from build123d import *

# Parameters (mm, degrees)
F0_R         = 15
F1_DEPTH     = 74
F2_R         = 15
F2_R_2       = 9.975
F3_DEPTH     = 3
F4_R         = 15
F4_R_2       = 10.0175
F5_DEPTH     = 22
F6_R         = 15
F6_R_2       = 7.5
F7_DEPTH     = 19
F8_SIZE2     = 1
F8_SIZE      = 1
F12_DEPTH    = 26.5
F13_T1_DEPTH = 5
F16_DEPTH    = 3


# Not quite as in the source:
# - a fillet or chamfer that OpenCascade refuses, or shapes differently, is made with other operations: its cross-section is extruded or revolved along the edge and cut away or added


with BuildPart() as f1:
    # F0 (on Front) → F1 (new body)
    with BuildSketch(Plane.XZ):
        Circle(F0_R)
    extrude(amount=F1_DEPTH)

    # F2 (on face) → F3 (cut)
    with BuildSketch(Plane.XZ.offset(74)):
        Circle(F2_R)
        Circle(F2_R_2, mode=Mode.SUBTRACT)
    extrude(amount=-F3_DEPTH, mode=Mode.SUBTRACT)

    # F4 (on face) → F5 (cut)
    with BuildSketch(Plane.XZ.offset(71)):
        Circle(F4_R)
        Circle(F4_R_2, mode=Mode.SUBTRACT)
    extrude(amount=-F5_DEPTH, mode=Mode.SUBTRACT)

    # F6 (on Front) → F7 (cut)
    with BuildSketch(Plane.XZ):
        Circle(F6_R)
        Circle(F6_R_2, mode=Mode.SUBTRACT)
    extrude(amount=F7_DEPTH, mode=Mode.SUBTRACT)

    # F8
    f8_edges = [f1.edges().sort_by_distance(p)[0] for p in [
        (-7.5, 0, 0),
        (-9.975, -74, 0),
    ]]
    chamfer(f8_edges, length=F8_SIZE, length2=F8_SIZE2)

    # F9 (on Right) → F10 (revolve, cut)
    with BuildSketch(Plane.YZ):
        Polygon((-26.5, 15), (-19, 7.5), (-19, 15), align=None)
    revolve(axis=Axis((0, -22.75, 0), (0, 1, 0)), mode=Mode.SUBTRACT)

    # F11 (on face) → F12 (cut)
    with BuildSketch(Plane.XZ.offset(74)):
        with BuildLine():
            Line((-2.5, 14.7901994577), (-2.5, 10.0175))
            Line((-2.5, 10.0175), (-2.5, 9.0175))
            Line((-2.5, 9.0175), (0, 9.0175))
            Line((0, 9.0175), (2.5, 9.0175))
            Line((2.5, 9.0175), (2.5, 10.0175))
            Line((2.5, 10.0175), (2.5, 14.7901994577))
            ThreePointArc((2.5, 14.7901994577), (0, 15), (-2.5, 14.7901994577))
        make_face()
    extrude(amount=-F12_DEPTH, mode=Mode.SUBTRACT)

    # F13: fillet of radius 2.5 on 1 edges, made by hand

    # F13_s2 → F13_t1 (join)
    with BuildSketch(Plane.YZ.offset(-2.5)):
        with BuildLine():
            add(Edge.make_bspline(
                [(-50, 9.0175), (-47.5, 9.0175), (-47.5, 11.5175)],
                knots=[0, 0, 0, 1, 1, 1], degree=2, weights=[1, 1, 1]))
            Line((-47.5, 11.5175), (-47.45, 11.5175))
            Line((-47.45, 11.5175), (-47.45, 8.9675))
            Line((-47.45, 8.9675), (-50, 8.9675))
            Line((-50, 8.9675), (-50, 9.0175))
        make_face()
    extrude(amount=F13_T1_DEPTH)

    # F15 (on offset) → F16 (cut)
    with BuildSketch(Plane.XY.offset(7.5)):
        with BuildLine():
            Line((2.5, -9), (2.5, -4))
            ThreePointArc((2.5, -4), (1.767766953, -2.232233047), (0, -1.5))
            ThreePointArc((0, -1.5), (-1.767766953, -2.232233047), (-2.5, -4))
            Line((-2.5, -4), (-2.5, -9))
            ThreePointArc((-2.5, -9), (-1.767766953, -10.767766953), (0, -11.5))
            ThreePointArc((0, -11.5), (1.767766953, -10.767766953), (2.5, -9))
        make_face()
    extrude(amount=-F16_DEPTH, mode=Mode.SUBTRACT)


solid = f1.part
Model file for the job. Use its own axes, mm. A direction names the side the tool comes from. Give positions to 0.01 mm unless a question says otherwise; leave off trailing zeros. Order: outer loops, then holes, each group sorted by start corner. A loop starts at its lowest first (then second) coordinate and runs counter-clockwise, first axis right, second up. Notation, with made-up numbers: M 6.5,-37.75 L 17.5,-37.75 A9 ccw 17.5,-22.75 Z; hole C 86,83 d10. An arc over 180 degrees is marked long. Put each result on its own line as item: value. Start each with the question number.
(1) Pull direction X, two halves, no side cores. Call faces 1 (the face through (-0.403, -72.014, -9.967)), 2 (the face through (0, -6, 4.5)), 3 (the face through (0, 0, 0)), 4 (the face through (2.5, -7, 6)): released by +X, released by -X, zero draft, split by the parting line, or undercut.
(2) Pin check, flat tips, straight feed: pin 1 Ø5 at (x, y) = (0.5, -52.5) entering from +Z; pin 2 Ø8 at (y, z) = (-65.5, 9.5) entering from -X; pin 3 Ø4.5 at (y, z) = (-62, 11.5) entering from +X. Stop position of each tip, or through.
(3) Band-saw the part on C-C on y = -38.5. Give the cut face in (x, z), then the cut area to 3 significant figures.
(4) Tool access for faces 5 (the face through (-0.41, -60.15, -10.01)), 6 (the face through (-2.5, -6, 6)), 7 (the face through (-1.63, -9.87, -7.32)), 8 (the face through (-2.5, -57.7, 9.4)), 9 (the face through (-3.252, -37.592, -14.643)): list every direction of +Z, -Z, +X, -X, +Y, -Y with a clear straight run to the whole face (end or side of a thin tool).
(5) Drill centre lines: L1, parallel to Z at x = -3, y = -8.5; L2, parallel to Y at x = -11, z = 6.5; L3, parallel to Z at x = -4.25, y = -59. Where is each one in solid material? Low to high. Write a range as [from, to].
(6) Band-saw the part on B-B on y = -67.5. Give the cut face in (x, z) (1 decimal).
Results below:
1. face 1: split by the parting line
1. face 2: undercut
1. face 3: zero draft
1. face 4: undercut
2. pin 1: stops at z = 9.7
2. pin 2: stops at x = -8.37
2. pin 3: stops at x = 3.85
3. outline: C 0,0 d30
3. area: 707 mm2
4. face 5: -Y
4. face 6: +Z
4. face 7: +Y
4. face 8: +Z, -Y
4. face 9: +Y, -Y
5. L1: z = [-6.87, 6.87]
5. L2: y = [-49, -24.28]
5. L3: z = [-9.07, 9.07]
6. outline: M -2.5,9 L -2.5,9.7 A10 ccw long 2.5,9.7 L 2.5,9 Z
